Part model, mm, in its own coordinate system. Round coordinates to 2 decimals unless told otherwise and drop trailing zeros. Loops run counter-clockwise (first coordinate to the right, second up) from the corner with the lowest first, then second, coordinate; pieces in that order, holes last.
1) Drop flat-ended pins along their axis: P1, Ø1, axis at x = 5, z = 0.5, coming from the +Y side; P2, Ø1, axis at x = -111, z = 1.5, coming from the -Y side; P3, Ø1, axis at x = -9.5, z = 2.5, coming from the +Y side. Give the stop position or say it passes through.
2) Band-saw the part on C-C, the plane y = 19.5. Write the cut outline in (x, z), then the cut area to 3 significant figures.
3) Band-saw the part on A-A, the plane x = 15. Write the cut outline in (y, z).
4) Probe line 1 (Y direction, x = -20, z = 2.4); line 2 (Y direction, x = 17, z = 1.6); line 3 (X direction, y = 12, z = 2). List the from-to ranges inside material, lowest first.
5) Band-saw the part on D-D, the plane x = -70.5. Write the cut outline in (y, z), then the cut area to 3 significant figures.
6) Band-saw the part on B-B, the plane z = 0.9. Write the cut outline in (x, y) (3 decimals), then the cut area to 3 significant figures.
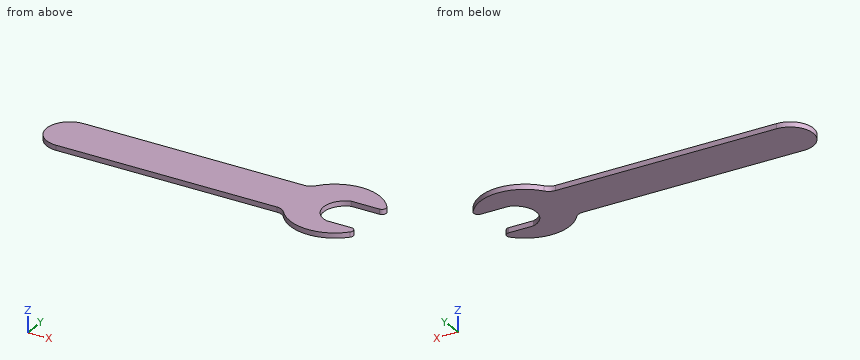
from build123d import *

# Parameters (mm, degrees)
F1_DEPTH = 2.8194


with BuildPart() as f1:
    # F0 (on Top) → F1 (new body)
    with BuildSketch(Plane.XY):
        with BuildLine():
            ThreePointArc((-5.911858, 28.195099), (-8.135546, 26.385217), (-10.928661, 25.737936))
            Line((-10.928661, 25.737936), (-134.269512, 25.737936))
            ThreePointArc((-134.269512, 25.737936), (-147.13848, 12.868968), (-134.269512, 0))
            Line((-134.269512, 0), (-10.928661, 0))
            ThreePointArc((-10.928661, 0), (-8.135546, -0.647281), (-5.911858, -2.457163))
            ThreePointArc((-5.911858, -2.457163), (12.871345, -12.112285), (32.345354, -3.939582))
            ThreePointArc((32.345354, -3.939582), (32.769998, -1.313703), (30.54071, 0.137446))
            Line((30.54071, 0.137446), (16.633371, 0.137446))
            ThreePointArc((16.633371, 0.137446), (8.182531, 11.737446), (16.633371, 23.337446))
            Line((16.633371, 23.337446), (32.345354, 23.337446))
            ThreePointArc((32.345354, 23.337446), (34.506755, 24.647631), (34.344997, 27.169945))
            ThreePointArc((34.344997, 27.169945), (14.475764, 37.860866), (-5.911858, 28.195099))
        make_face()
    extrude(amount=F1_DEPTH)


solid = f1.part
Reported:
1. P1: stops at y = 36.44
1. P2: stops at y = 0
1. P3: stops at y = 26.04
2. outline: (-145.3, 0) - (10.97, 0) - (10.97, 2.82) - (-145.3, 2.82) - close
2. area: 441 mm2
3. outline: (-12.1, 0) - (0.8, 0) - (0.8, 2.82) - (-12.1, 2.82) - close; (22.68, 0) - (37.84, 0) - (37.84, 2.82) - (22.68, 2.82) - close
4. line 1: y = 0 to 25.74
4. line 2: y = -11.93 to 0.14, 23.34 to 37.67
4. line 3: x = -147.11 to 8.19
5. outline: (0, 0) - (25.74, 0) - (25.74, 2.82) - (0, 2.82) - close
5. area: 72.6 mm2
6. outline: (-134.27, 0) - (-10.929, 0) arc R6.35 cw to (-5.912, -2.457) arc R25 ccw to (32.345, -3.94) arc R2.438 ccw to (30.541, 0.137) - (16.633, 0.137) arc R12.187 cw to (16.633, 23.337) - (32.345, 23.337) arc R2.438 ccw to (34.345, 27.17) arc R25 ccw to (-5.912, 28.195) arc R6.35 cw to (-10.929, 25.738) - (-134.27, 25.738) arc R12.869 ccw to start
6. area: 4,780 mm2
